Here's how the part is built. I have some questions about the finished solid (model axes, mm). Face numbers are marked on the shaded views. Coordinates: 2 decimals unless noted, no trailing zeros. Write each loop counter-clockwise with the first axis right and the second up, starting at its lowest first coordinate (ties: lowest second). Pieces come first, ordered by that corner, then holes.
Item 1: I want a section at A-A (z = 1.35). Please give me the cut outline in (x, y).
Item 2: If we mould it in two halves opening along X, with no side actions, what happens to the marked faces 1, 2 and 3? For each: pulls with the +X half, pulls with the -X half, needs draft (parallel to the pull), parting line crosses it, or undercut.
Item 3: Please list where these lines run through material, in increasing order: line 1 (Y direction, x = 0, z = 3.75); line 2 (X direction, y = -7.5, z = 3.25); line 3 (X direction, y = -3.5, z = 2.2).
Item 4: I want a section at C-C (y = -10). Please give me the cut outline in (x, z).
Item 5: I want a section at B-B (x = 26). Please give me the cut outline in (y, z), and give its area (3 significant figures).
Item 6: I'm going to push flat-ended pins straight in: P1, Ø3, axis at y = 24.5, z = 3, coming from the +X side; P2, Ø3, axis at y = 15.5, z = 2, coming from the +X side. Where does each tip first touch, or does it pass through?
Item 7: I want a section at D-D (x = 2). Please give me the cut outline in (y, z), and give its area (3 significant figures).
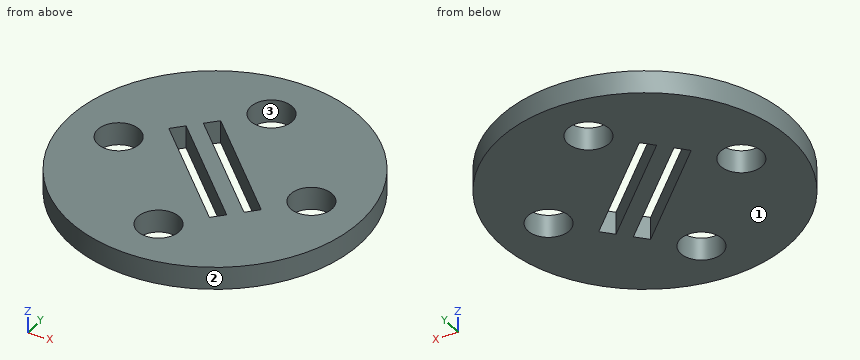
from build123d import *

# Parameters (mm, degrees)
MODEL_R             = 38.5
MODEL_R_2           = 5.5
BOSS_EXTRUDE1_DEPTH = 6


with BuildPart() as part:
    # Model → Boss-Extrude1 (new body)
    with BuildSketch(Plane.XY):
        Circle(MODEL_R)
        with Locations((-25, 0)):
            Circle(MODEL_R_2, mode=Mode.SUBTRACT)
        with Locations((0, 25)):
            Circle(MODEL_R_2, mode=Mode.SUBTRACT)
        with Locations((0, -25)):
            Circle(MODEL_R_2, mode=Mode.SUBTRACT)
        with Locations((25, 0)):
            Circle(MODEL_R_2, mode=Mode.SUBTRACT)
        Polygon((-16.970562748, 8.485281374), (-14.142135624, 11.313708499), (11.313708499, -14.142135624), (8.485281374, -16.970562748), align=None, mode=Mode.SUBTRACT)
        Polygon((-11.313708499, 14.142135624), (14.142135624, -11.313708499), (16.970562748, -8.485281374), (-8.485281374, 16.970562748), align=None, mode=Mode.SUBTRACT)
    extrude(amount=BOSS_EXTRUDE1_DEPTH)


solid = part.part
Answer:
1. outline: circle Ø77 at (0, 0); hole circle Ø11 at (-25, 0); hole (-16.97, 8.49) - (8.49, -16.97) - (11.31, -14.14) - (-14.14, 11.31) - close; hole (-11.31, 14.14) - (14.14, -11.31) - (16.97, -8.49) - (-8.49, 16.97) - close; hole circle Ø11 at (0, -25); hole circle Ø11 at (0, 25); hole circle Ø11 at (25, 0)
2. face 1: needs draft
2. face 2: parting line crosses it
2. face 3: undercut
3. line 1: y = -38.5 to -30.5, -19.5 to -8.49, -2.83 to 2.83, 8.49 to 19.5, 30.5 to 38.5
3. line 2: x = -37.76 to -0.99, 4.67 to 10.33, 15.99 to 37.76
3. line 3: x = -38.34 to -29.24, -20.76 to -4.99, 0.67 to 6.33, 11.99 to 20.76, 29.24 to 38.34
4. outline: (-37.18, 0) - (1.51, 0) - (1.51, 6) - (-37.18, 6) - close; (7.17, 0) - (12.83, 0) - (12.83, 6) - (7.17, 6) - close; (15.46, 0) - (37.18, 0) - (37.18, 6) - (15.46, 6) - close
5. outline: (-28.39, 0) - (-5.41, 0) - (-5.41, 6) - (-28.39, 6) - close; (5.41, 0) - (28.39, 0) - (28.39, 6) - (5.41, 6) - close
5. area: 276 mm2
6. P1: stops at x = 30.87
6. P2: stops at x = 35.86
7. outline: (-38.45, 0) - (-30.12, 0) - (-30.12, 6) - (-38.45, 6) - close; (-19.88, 0) - (-10.49, 0) - (-10.49, 6) - (-19.88, 6) - close; (-4.83, 0) - (0.83, 0) - (0.83, 6) - (-4.83, 6) - close; (6.49, 0) - (19.88, 0) - (19.88, 6) - (6.49, 6) - close; (30.12, 0) - (38.45, 0) - (38.45, 6) - (30.12, 6) - close
7. area: 271 mm2
